Can you work these out from the model? Positions are in its coordinate system, mm. Face numbers are marked on the shaded views. A direction names the side the tool comes from. Coordinates: 2 decimals unless noted, no trailing zeros. Write each loop counter-clockwise with the first axis right and the second up, starting at its lowest first coordinate (ties: lowest second). Pieces come first, ordered by that corner, then holes. Notation, with made-up numbers: (3, 8) - (57, 8) arc R31 ccw to (57, 34) - close; hole circle Ø7 at (43.5, 64). An arc over 180 degrees is marked (long way). One line per question, with ' | ' between items. Start each with the question number.
from build123d import *

# Parameters (mm, degrees)
F1_DEPTH = 50.8
F2_W     = 106.4794771373
F2_H     = 20.7544723526
F3_DEPTH = 85.852


with BuildPart() as f1:
    # F0 (on Top) → F1 (new body)
    with BuildSketch(Plane.XY):
        with BuildLine():
            Line((63.5, -21.5948767427), (63.5, 21.5948767427))
            ThreePointArc((63.5, 21.5948767427), (47.4267261232, 47.4267261232), (21.5948767427, 63.5))
            Line((21.5948767427, 63.5), (-21.5948767427, 63.5))
            ThreePointArc((-21.5948767427, 63.5), (-47.4267261232, 47.4267261232), (-63.5, 21.5948767427))
            Line((-63.5, 21.5948767427), (-63.5, -21.5948767427))
            ThreePointArc((-63.5, -21.5948767427), (-47.4267261232, -47.4267261232), (-21.5948767427, -63.5))
            Line((-21.5948767427, -63.5), (21.5948767427, -63.5))
            ThreePointArc((21.5948767427, -63.5), (47.4267261232, -47.4267261232), (63.5, -21.5948767427))
        make_face()
    extrude(amount=F1_DEPTH)

    # F2 (on Front) → F3 (cut, symmetric)
    with BuildSketch(Plane.XZ):
        with Locations((-10.3772375733, 25.2663153224)):
            Rectangle(F2_W, F2_H)
    extrude(amount=F3_DEPTH, both=True, mode=Mode.SUBTRACT)


solid = f1.part
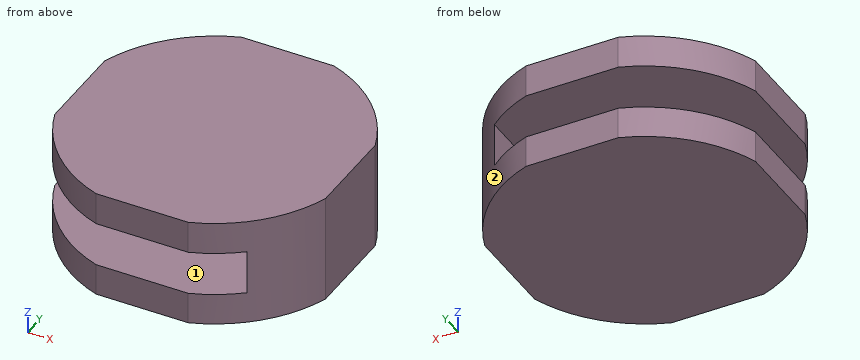
(1) If I drill on probe 1 along Z at (x, y) = (38, 35); probe 2 along X at (y, z) = (2, 29); probe 3 along Y at (x, z) = (48, 18.5), over which ranges is the centre line in solid material (lowest first)?
(2) If we section it at B-B on z = 7: List the corners of the cut face in (x, y) for me, plus the area to 3 significant figures.
(3) Which directions (+Z, -Z, +X, -X, +Y, -Y) give clear straight access to the entire face, cutting with the end or side of a thin tool? Please do the marked faces 1 and 2.
(4) If we section it at D-D on x = 52.5: List the corners of the cut face in (y, z) for me.
(5) If we section it at C-C on y = 6.5: List the corners of the cut face in (x, z) for me.
(6) If we section it at A-A on x = -11: List the corners of the cut face in (y, z) for me, plus the area to 3 significant figures.
(7) I'm going to push flat-ended pins straight in: pin 1 (10 mm diameter, centred on x = -1, y = -34.5, fed in from -Z); pin 2 (3 mm diameter, centred on x = 39.5, z = 37.5, fed in from -Y); pin 3 (1.5 mm diameter, centred on x = 43.5, z = 21.5, fed in from +Y); pin 4 (3 mm diameter, centred on y = 40.5, z = 28, fed in from -X). Where does each tip first touch, or does it pass through?
Values:
1) probe 1: 0 to 14.89, 35.64 to 50.8 | probe 2: 42.86 to 63.5 | probe 3: -46.85 to 46.85
2) outline: (-63.5, -21.59) arc R67.07 ccw to (-21.59, -63.5) - (21.59, -63.5) arc R67.07 ccw to (63.5, -21.59) - (63.5, 21.59) arc R67.07 ccw to (21.59, 63.5) - (-21.59, 63.5) arc R67.07 ccw to (-63.5, 21.59) - close | area: 13,700 mm2
3) face 1: -X, +Y, -Y | face 2: +Z, -Z, +X, +Y
4) outline: (-41.74, 0) - (41.74, 0) - (41.74, 50.8) - (-41.74, 50.8) - close
5) outline: (-63.5, 0) - (63.5, 0) - (63.5, 50.8) - (-63.5, 50.8) - (-63.5, 35.64) - (42.86, 35.64) - (42.86, 14.89) - (-63.5, 14.89) - close
6) outline: (-63.5, 0) - (63.5, 0) - (63.5, 14.89) - (-63.5, 14.89) - close; (-63.5, 35.64) - (63.5, 35.64) - (63.5, 50.8) - (-63.5, 50.8) - close | area: 3,820 mm2
7) pin 1: z = 0 | pin 2: y = -55.27 | pin 3: y = 51.59 | pin 4: x = 42.86
